```python
from build123d import *

# Parameters (mm, degrees)
F1_DEPTH = 25.4
F3_DEPTH = 25.4
F4_DEPTH = 25.4


with BuildPart() as f1:
    # F0 (on Front) → F1 (new body)
    with BuildSketch(Plane.XZ):
        Polygon((12.8309270367, 36.0182486475), (0, 36.0182486475), (0, 0), (51.5070110559, 0), (51.5070110559, 36.0182486475), (39.9591773748, 36.0182486475), (39.9591773748, 20.9877323359), (12.8309270367, 20.9877323359), align=None)
    extrude(amount=F1_DEPTH)

    # F2 (on face) → F3 (join)
    with BuildSketch(Plane.YZ.offset(51.5070110559)):
        Polygon((-18.5131952167, 29.4194854796), (-18.5131952167, 36.0182486475), (-25.4, 36.0182486475), (-25.4, 0), (0, 0), (0, 36.0182486475), (-7.1486602537, 36.0182486475), (-7.1486602537, 29.4194854796), align=None)
    extrude(amount=F3_DEPTH)

    # F4 (cut): a face of the model
    f4_faces = [f1.faces().sort_by_distance(p)[0] for p in [
        (51.5070110559, -12.8309277352, 32.7188670635),
    ]]
    extrude(f4_faces, amount=-F4_DEPTH, mode=Mode.SUBTRACT)


solid = f1.part
```
Input: part model. Units: mm. Frame: model coordinates. A direction names the side the tool comes from. Coordinates: 2 decimals unless noted, no trailing zeros. Loops run counter-clockwise (first coordinate to the right, second up) from the corner with the lowest first, then second, coordinate; pieces in that order, holes last.
Q1. Mould query, pull axis X, two halves, no side actions, for faces 1 (the flat face through (58, -4, 36.018)), 2 (the flat face through (76.907, -13, 18)), 3 (the flat face through (0, -13, 18)), 4 (the flat face through (39.959, -13, 27)). Classes: +X half, -X half, draft (parallel to the pull), parting line (faces both ways), or undercut.
Results are:
face 1: draft
face 2: +X half
face 3: -X half
face 4: undercut
Q2. Set-up query: faces 5 (the flat face through (58, -22, 36.018)), 6 (the flat face through (27, -13, 20.988)), 7 (the flat face through (58, -13, 29.419)). Return all of +Z, -Z, +X, -X, +Y, -Y with unobstructed straight access to the full face (end or side cutting, diameter ignored); none if empty.
Results are:
face 5: +Z, +X, -X, +Y, -Y
face 6: +Z, +Y, -Y
face 7: +Z, +X
Q3. Section A-A, the plane z = 28. Return the cut outline in (x, y).
Results are:
outline: (0, -25.4) - (12.83, -25.4) - (12.83, 0) - (0, 0) - close; (39.96, -25.4) - (76.91, -25.4) - (76.91, 0) - (39.96, 0) - close
Q4. Section C-C, the plane z = 33.5. Return the cut outline in (x, y).
Results are:
outline: (0, -25.4) - (12.83, -25.4) - (12.83, 0) - (0, 0) - close; (39.96, -25.4) - (76.91, -25.4) - (76.91, -18.51) - (39.96, -18.51) - close; (39.96, -7.15) - (76.91, -7.15) - (76.91, 0) - (39.96, 0) - close
Q5. Section D-D, the plane x = 68. Return the cut outline in (y, z), and give its area (3 significant figures).
Results are:
outline: (-25.4, 0) - (0, 0) - (0, 36.02) - (-7.15, 36.02) - (-7.15, 29.42) - (-18.51, 29.42) - (-18.51, 36.02) - (-25.4, 36.02) - close
area: 840 mm2
Q6. Line query: line 1 along X through (y, z) = (-2.75, 27.5); line 2 along Z through (x, y) = (62, -10.25); line 3 along X through (y, z) = (-13, 35.5). Output: solid intervals per line, ascending.
Results are:
line 1: x = 0 to 12.83, 39.96 to 76.91
line 2: z = 0 to 29.42
line 3: x = 0 to 12.83
Q7. Contact query for flat-ended pins moving along their axis: pin 1 (1.5 mm diameter, centred on x = 36, y = -9.5, fed in from +Z); pin 2 (4 mm diameter, centred on x = 58.5, y = -14.5, fed in from +Z). Output: stop coordinate, or through.
Results are:
pin 1: stops at z = 20.99
pin 2: stops at z = 29.42
Q8. Section B-B, the plane y = -10.75. Return the cut outline in (x, z).
Results are:
outline: (0, 0) - (76.91, 0) - (76.91, 29.42) - (39.96, 29.42) - (39.96, 20.99) - (12.83, 20.99) - (12.83, 36.02) - (0, 36.02) - close
